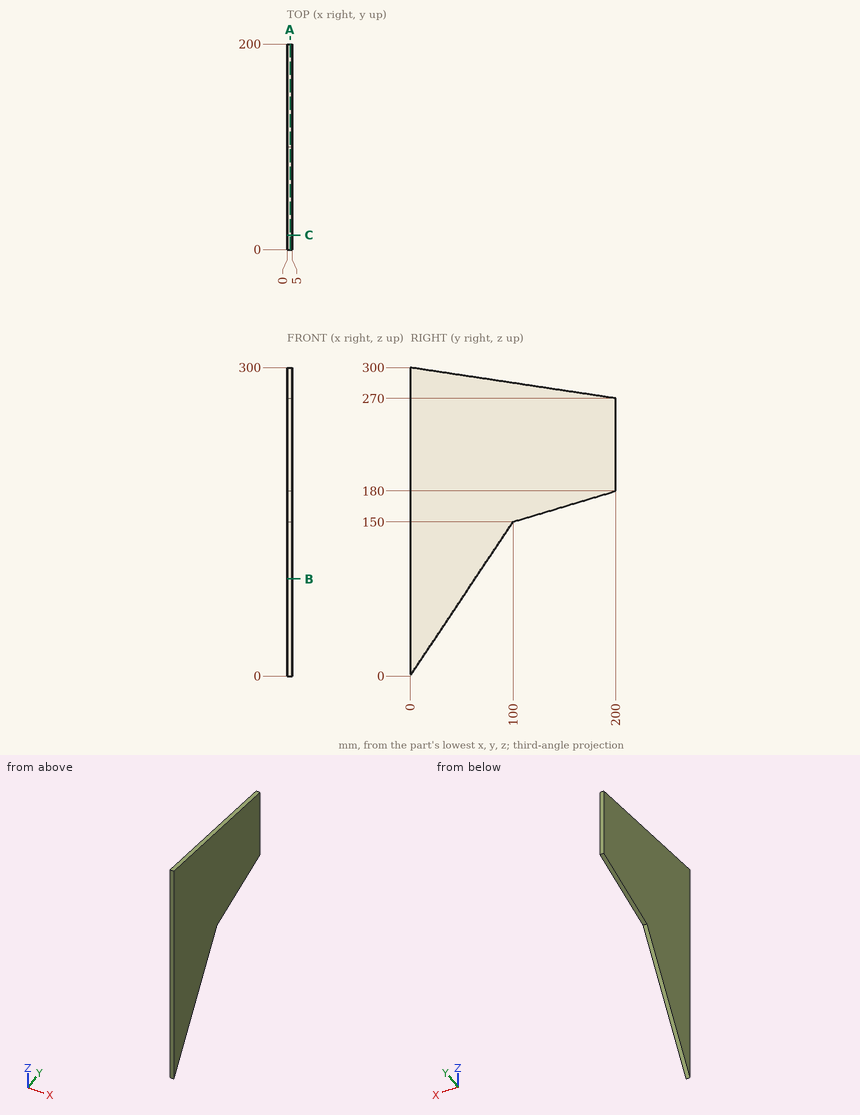
Check sheet for the drawn part. Datum: minimum x, y, z corner. Units: mm. Round coordinates to 2 decimals unless told otherwise and drop trailing zeros. Loops run counter-clockwise (first coordinate to the right, second up) from the corner with the lowest first, then second, coordinate; pieces in that order, holes last. Notation, with made-up numbers: M 39,79 L 96,79 A31 cw 96,117 Z; hole C 38.5,82 d6. An arc over 180 degrees is marked long. One line per question, with ' | ' between items. Start each with the question number.
Item 1: Scan lines: probe 1 along Z at (x, y) = (0.35, 13.5) (3 decimals); probe 2 along Z at (x, y) = (4.1, 82); probe 3 along Y at (x, z) = (0.2, 146.5). Record each from-to range of solid material in increasing order.
Item 2: Section check B-B (z = 94.5). Record the boundary of the cut face in (x, y).
Item 3: Gauge pin test, flat ends, axial feed: pin 1 Ø3 at (x, y) = (2, 91.5) entering from +Z; pin 2 Ø1.5 at (x, y) = (3, 53.5) entering from -Z (3 decimals); pin 3 Ø2 at (x, y) = (3, 152) entering from -Z. Record the tip position at first contact, or that the pin passes through.
Item 4: Section check C-C (y = 14). Record the boundary of the cut face in (x, z).
Item 5: Section check A-A (x = 2.85). Record the boundary of the cut face in (y, z).
Worked out:
1) probe 1: 20.25 to 297.975 | probe 2: 123 to 287.7 | probe 3: 0 to 97.67
2) outline: M 0,0 L 5,0 L 5,63 L 0,63 Z
3) pin 1: z = 286.5 | pin 2: z = 79.125 | pin 3: z = 165.3
4) outline: M 0,21 L 5,21 L 5,297.9 L 0,297.9 Z
5) outline: M 0,0 L 100,150 L 200,180 L 200,270 L 0,300 Z
